Verification items for this drawing (mm, ordinates from the low corner). A direction names the side the tool comes from. Coordinates: 2 decimals unless noted, no trailing zeros. Loops run counter-clockwise (first coordinate to the right, second up) from the corner with the lowest first, then second, coordinate; pieces in that order, holes last. Notation, with made-up numbers: M 52.25,48.5 L 95.25,48.5 A23 cw 95.25,70.5 Z; hole C -23,-10 d8. An arc over 180 degrees is marked long. Write each question's results on one line, items separated by ' | '. Start each with the question number.
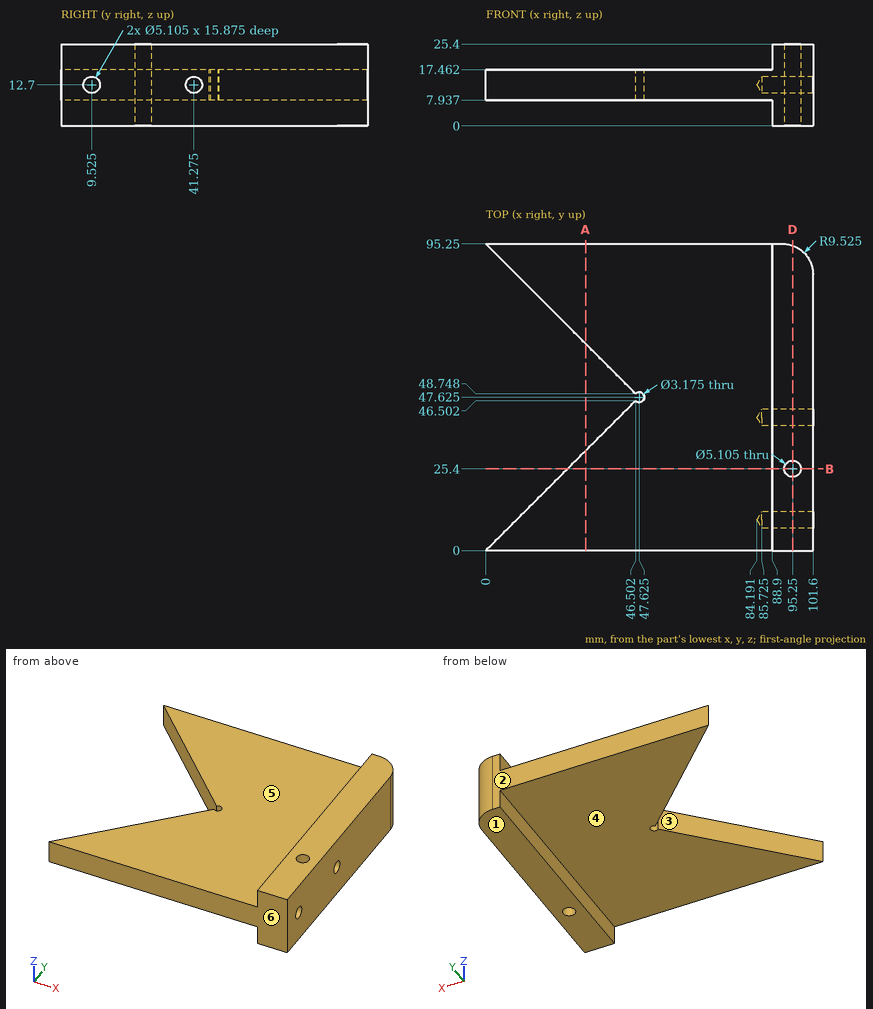
Item 1: Release check for a two-part mould opening along Y. For the marked faces 1, 2 and 3 record: +Y half, -Y half, draft (parallel to the pull), parting line (faces both ways), or undercut.
Item 2: Section check A-A (x = 31). Record the cut outline in (y, z).
Item 3: Tool access check on the marked faces 4, 5 and 6. Record the directions out of +Z, -Z, +X, -X, +Y, -Y that give a thin tool (end or side, any length) a straight path to the whole face; none if there is none.
Item 4: Thickness scan on line 1 (Y direction, x = 90.25, z = 12.7); line 2 (Y direction, x = 94, z = 12.7) (1 decimal); line 3 (X direction, y = 52, z = 20). Record the ranges inside material, lowest first.
Item 5: Section check B-B (y = 25.4). Record the cut outline in (x, z).
Item 6: Section check D-D (x = 95.25). Record the cut outline in (y, z) (1 decimal).
Item 7: Depth check by flat-ended pin: P1, Ø8, axis at x = 12, y = 18, coming from the -Z side; P2, Ø8, axis at x = 70, y = 75.5, coming from the -Z side; P3, Ø6, axis at y = 41.275, z = 12.7, coming from the -X side (1 decimal); P4, Ø8.5, axis at y = 41.5, z = 23.5, coming from the -X side. Enter the tip coordinate at first touch or a pass-through.
Computed values:
1) face 1: draft | face 2: +Y half | face 3: undercut
2) outline: M 0,7.94 L 31,7.94 L 31,17.46 L 0,17.46 Z; M 64.25,7.94 L 95.25,7.94 L 95.25,17.46 L 64.25,17.46 Z
3) face 4: -Z, -X, +Y, -Y | face 5: +Z, -X, +Y, -Y | face 6: +Z, -Z, +X, -X, -Y
4) line 1: y = 0 to 6.97, 12.08 to 38.72, 43.83 to 95.25 | line 2: y = 0 to 7, 12.1 to 23.2, 27.6 to 38.7, 43.8 to 95.1 | line 3: x = 88.9 to 101.6
5) outline: M 25.4,7.94 L 88.9,7.94 L 88.9,0 L 92.7,0 L 92.7,25.4 L 88.9,25.4 L 88.9,17.46 L 25.4,17.46 Z; M 97.8,0 L 101.6,0 L 101.6,25.4 L 97.8,25.4 Z
6) outline: M 0,0 L 22.8,0 L 22.8,25.4 L 0,25.4 Z; M 28,0 L 94.7,0 L 94.7,25.4 L 28,25.4 Z; hole C 9.5,12.7 d5.1; hole C 41.3,12.7 d5.1
7) P1: passes through | P2: stops at z = 7.94 | P3: stops at x = 38.3 | P4: stops at x = 88.9
